Check sheet for the modelled part. Datum: model origin and axes. Units: mm. A direction names the side the tool comes from. Give positions to 0.01 mm unless a question says otherwise; leave off trailing zeros. Write each loop counter-clockwise with the first axis right and the second up, starting at its lowest first coordinate (ties: lowest second). Pieces come first, ordered by that corner, then holes. Notation, with made-up numbers: M 85,45 L 117,45 A8 ccw 117,60 Z; hole C -8,29.25 d11. An arc over 180 degrees is marked long. Write item = value, one per line. Start each with the question number.
1) Sectioned sample at B-B, the plane z = 0.75. Record the cut outline in (x, y), then the cut area to 3 significant figures.
2) Set-up check for faces 4 (the face through (0, -14, 2)), 5 (the face through (4.9, 0, -3)), 6 (the face through (3.199, 15.715, 2.894)): record each of +Z, -Z, +X, -X, +Y, -Y from which the full face is reachable in a straight line by a thin tool's end or side.
3) Gauge pin test, flat ends, axial feed: pin 1 (2 mm diameter, centred on y = 0.5, z = 3, fed in from +X); pin 2 (1.4 mm diameter, centred on x = -0.5, z = 2.5, fed in from +Y); pin 3 (3 mm diameter, centred on x = 0, y = -3.5, fed in from +Z); pin 4 (0.9 mm diameter, centred on x = 0, z = 3, fed in from -Y). Record the tip position at first contact, or that the pin passes through.
4) Draft check along Y on faces 1 (the face through (-3.215, 15.699, 2.894)), 2 (the face through (0, -17.7, -3)), 3 (the face through (0, -16, 3)). Enter one of: pulls with the +Y half, pulls with the -Y half, needs draft (parallel to the pull), parting line crosses it, or undercut.
5) Sectioned sample at A-A, the plane y = 11.5. Record the cut outline in (x, z).
6) Scan lines: L1, parallel to X at y = -11, z = -0.5; L2, parallel to Y at x = 4, z = -2.5; L3, parallel to Y at x = -1.5, z = 0.5. Record each from-to range of solid material in increasing order.
7) Sectioned sample at D-D, the plane x = 3. Record the cut outline in (y, z).
8) Sectioned sample at C-C, the plane z = 3.25. Record the cut outline in (x, y).
from build123d import *

# Parameters (mm, degrees)
SKETCH1_W      = 14
SKETCH1_H      = 40
SKETCH1_W_2    = 3.5
SKETCH1_H_2    = 28
EXTRUDE1_DEPTH = 1.5
SKETCH2_W      = 7
SKETCH2_H      = 32
SKETCH2_W_2    = 3.5
SKETCH2_H_2    = 28
EXTRUDE2_DEPTH = 2.75
SKETCH3_W      = 14
SKETCH3_H      = 40
SKETCH3_W_2    = 9.8
SKETCH3_H_2    = 35.4
EXTRUDE3_DEPTH = 6
FILLET1_R      = 0.25
FILLET2_R      = 1


with BuildPart() as part:
    # Sketch1 → Extrude1 (new body)
    with BuildSketch(Plane.XY):
        Rectangle(SKETCH1_W, SKETCH1_H)
        Rectangle(SKETCH1_W_2, SKETCH1_H_2, mode=Mode.SUBTRACT)
    extrude(amount=EXTRUDE1_DEPTH)

    # Sketch2 → Extrude2 (add)
    with BuildSketch(Plane.XY.offset(1.5)):
        Rectangle(SKETCH2_W, SKETCH2_H)
        Rectangle(SKETCH2_W_2, SKETCH2_H_2, mode=Mode.SUBTRACT)
    extrude(amount=EXTRUDE2_DEPTH)

    # Sketch3 → Extrude3 (add)
    with BuildSketch(Plane(origin=(0, 0, 0), x_dir=(-1, 0, 0), z_dir=(0, 0, -1))):
        Rectangle(SKETCH3_W, SKETCH3_H)
        Rectangle(SKETCH3_W_2, SKETCH3_H_2, mode=Mode.SUBTRACT)
    extrude(amount=EXTRUDE3_DEPTH)

    # Fillet1
    fillet1_edges = [part.edges().sort_by_distance(p)[0] for p in [
        (1.75, -14, 2.125),
        (1.75, 14, 2.125),
        (-1.75, 14, 2.125),
        (-1.75, -14, 2.125),
        (-4.9, 17.7, -3),
        (4.9, 17.7, -3),
        (4.9, -17.7, -3),
        (-4.9, -17.7, -3),
    ]]
    fillet(fillet1_edges, radius=FILLET1_R)

    # Fillet2
    fillet2_edges = [part.edges().sort_by_distance(p)[0] for p in [
        (3.5, -16, 2.875),
        (3.5, 16, 2.875),
        (-3.5, 16, 2.875),
        (-3.5, -16, 2.875),
        (7, -20, -2.25),
        (-7, -20, -2.25),
        (-7, 20, -2.25),
        (7, 20, -2.25),
    ]]
    fillet(fillet2_edges, radius=FILLET2_R)


solid = part.part
Data:
q1.outline = M -7,-19 A1 ccw -6,-20 L 6,-20 A1 ccw 7,-19 L 7,19 A1 ccw 6,20 L -6,20 A1 ccw -7,19 Z; hole M -1.75,-13.75 A0.25 ccw -1.5,-14 L 1.5,-14 A0.25 ccw 1.75,-13.75 L 1.75,13.75 A0.25 ccw 1.5,14 L -1.5,14 A0.25 ccw -1.75,13.75 Z
q1.area = 461 mm2
q2.face_4 = +Z, -Z
q2.face_5 = -Z
q2.face_6 = +Z, +X, +Y
q3.pin_1 = 3.5
q3.pin_2 = 16
q3.pin_3 = through
q3.pin_4 = -16
q4.face_1 = pulls with the +Y half
q4.face_2 = undercut
q4.face_3 = pulls with the -Y half
q5.outline = M -7,-6 L -4.9,-6 L -4.9,0 L -1.75,0 L -1.75,4.25 L -3.5,4.25 L -3.5,1.5 L -7,1.5 Z; M 1.75,0 L 4.9,0 L 4.9,-6 L 7,-6 L 7,1.5 L 3.5,1.5 L 3.5,4.25 L 1.75,4.25 Z
q6.L1 = -7 to -4.9, 4.9 to 7
q6.L2 = -20 to -17.7, 17.7 to 20
q6.L3 = -20 to -14, 14 to 20
q7.outline = M -20,-6 L -17.7,-6 L -17.7,0 L 17.7,0 L 17.7,-6 L 20,-6 L 20,1.5 L 15.87,1.5 L 15.87,4.25 L -15.87,4.25 L -15.87,1.5 L -20,1.5 Z
q8.outline = M -3.5,-15 A1 ccw -2.5,-16 L 2.5,-16 A1 ccw 3.5,-15 L 3.5,15 A1 ccw 2.5,16 L -2.5,16 A1 ccw -3.5,15 Z; hole M -1.75,-13.75 A0.25 ccw -1.5,-14 L 1.5,-14 A0.25 ccw 1.75,-13.75 L 1.75,13.75 A0.25 ccw 1.5,14 L -1.5,14 A0.25 ccw -1.75,13.75 Z
